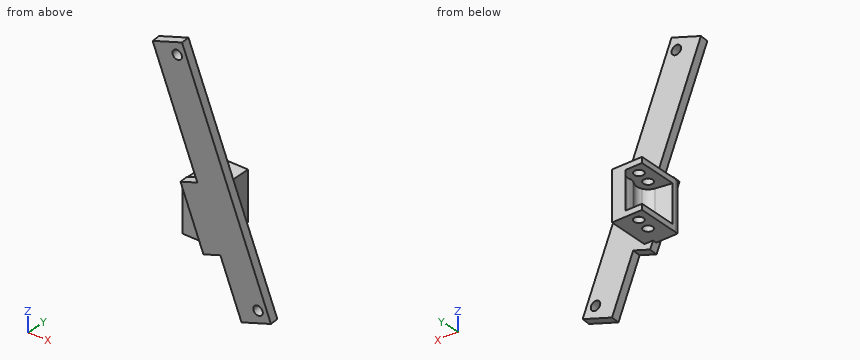
from build123d import *

# Parameters (mm, degrees)
BOSS_EXTRUDE1_DEPTH = 29.21
SKETCH2_R           = 3.175
BOSS_EXTRUDE2_DEPTH = 3.81
SKETCH3_R           = 3.175
BOSS_EXTRUDE3_DEPTH = 3.81
SKETCH4_R           = 3.175
BOSS_EXTRUDE4_DEPTH = 5.588
BOSS_EXTRUDE5_DEPTH = 33.02


with BuildPart() as part:
    # Sketch1 → Boss-Extrude1 (new body)
    with BuildSketch(Plane.XY):
        with BuildLine():
            Line((468.75530918, 278.776071532), (459.631228606, 278.776071532))
            ThreePointArc((459.631228606, 278.776071532), (460.543620658, 278.201967285), (461.366897066, 277.506071532))
            ThreePointArc((461.366897066, 277.506071532), (463.397272377, 274.114329254), (463.477224231, 270.162121354))
            ThreePointArc((463.477224231, 270.162121354), (463.399405765, 268.135304283), (464.120754615, 266.239598875))
            ThreePointArc((464.120754615, 266.239598875), (465.307742726, 262.469481888), (464.467858916, 258.607187485))
            ThreePointArc((464.467858916, 258.607187485), (462.151375158, 255.897407535), (458.862647092, 254.521445295))
            Line((458.862647092, 254.521445295), (448.43530918, 252.810420021))
            Line((448.43530918, 252.810420021), (448.43530918, 250.486101833))
            Line((448.43530918, 250.486101833), (468.75530918, 250.486101833))
            Line((468.75530918, 250.486101833), (468.75530918, 278.776071532))
        make_face()
    extrude(amount=-BOSS_EXTRUDE1_DEPTH)

    # Sketch2 → Boss-Extrude2 (add)
    with BuildSketch(Plane.XY):
        Polygon((448.43530918, 252.810420021), (448.43530918, 278.776071532), (468.75530918, 278.776071532), (468.75530918, 250.486101833), (448.43530918, 250.486101833), align=None)
        with Locations(Location((455.996603091, 271.987703521, 0), (0, 0, 180))):
            Circle(SKETCH2_R, mode=Mode.SUBTRACT)
        with Locations(Location((457.615851502, 262.119672583, 0), (0, 0, 180))):
            Circle(SKETCH2_R, mode=Mode.SUBTRACT)
    extrude(amount=BOSS_EXTRUDE2_DEPTH)

    # Sketch3 → Boss-Extrude3 (add)
    # profile 1 of 3: a face of its own
    with BuildSketch(Plane(origin=(0, 0, -25.4), x_dir=(-1, 0, 0), z_dir=(0, 0, -1))):
        with BuildLine():
            Line((-464.467858916, 258.607187485), (-448.43530918, 255.976401177))
            Line((-448.43530918, 255.976401177), (-448.43530918, 275.384123064))
            Line((-448.43530918, 275.384123064), (-461.366897066, 277.506071532))
            ThreePointArc((-461.366897066, 277.506071532), (-463.397272377, 274.114329254), (-463.477224231, 270.162121354))
            ThreePointArc((-463.477224231, 270.162121354), (-463.399405765, 268.135304283), (-464.120754615, 266.239598875))
            ThreePointArc((-464.120754615, 266.239598875), (-465.307742726, 262.469481888), (-464.467858916, 258.607187485))
        make_face()
        with Locations((-457.615851502, 262.119672583)):
            Circle(SKETCH3_R, mode=Mode.SUBTRACT)
        with Locations((-455.996603091, 271.987703521)):
            Circle(SKETCH3_R, mode=Mode.SUBTRACT)
    # profile 2 of 3: a face of its own
    with BuildSketch(Plane(origin=(0, 0, -25.4), x_dir=(-1, 0, 0), z_dir=(0, 0, -1))):
        with BuildLine():
            Line((-458.862647092, 254.521445295), (-448.43530918, 252.810420021))
            Line((-448.43530918, 252.810420021), (-448.43530918, 255.976401177))
            Line((-448.43530918, 255.976401177), (-464.467858916, 258.607187485))
            ThreePointArc((-464.467858916, 258.607187485), (-462.151375158, 255.897407535), (-458.862647092, 254.521445295))
        make_face()
    # profile 3 of 3: a face of its own
    with BuildSketch(Plane(origin=(0, 0, -25.4), x_dir=(-1, 0, 0), z_dir=(0, 0, -1))):
        with BuildLine():
            Line((-461.366897066, 277.506071532), (-448.43530918, 275.384123064))
            Line((-448.43530918, 275.384123064), (-448.43530918, 278.776071532))
            Line((-448.43530918, 278.776071532), (-459.631228606, 278.776071532))
            ThreePointArc((-459.631228606, 278.776071532), (-460.543620658, 278.201967285), (-461.366897066, 277.506071532))
        make_face()
    extrude(amount=BOSS_EXTRUDE3_DEPTH)

    # Sketch4 → Boss-Extrude4 (add)
    with BuildSketch(Plane(origin=(-3.84203447, 241.841104975, 11.406767954), x_dir=(0.9998741117550617, 0.015849347043774307, 0.0007475562269394091), z_dir=(-0.015866967007794316, 0.9987637706378837, 0.04710806533037044))):
        Polygon((459.215763784, -85.500450968), (512.667124492, 73.389830794), (492.808231658, 80.070446074), (480.07788451, 42.228033485), (468.640206694, 46.075716527), (454.8306113, 5.025115122), (466.268289117, 1.17743208), (439.35687095, -78.819835688), align=None)
        with Locations(Location((455.674707496, -76.269609027, 0), (0, 0, 270))):
            Circle(SKETCH4_R, mode=Mode.SUBTRACT)
        with Locations(Location((504.266853595, 68.176101666, 0), (0, 0, 270))):
            Circle(SKETCH4_R, mode=Mode.SUBTRACT)
    extrude(amount=-BOSS_EXTRUDE4_DEPTH)

    # Sketch5 → Boss-Extrude5 (add)
    with BuildSketch(Plane.XY.offset(3.81)):
        Polygon((468.75530918, 250.486101833), (448.560469366, 250.486101833), (448.560469366, 248.52896412), (468.75530918, 248.393245925), align=None)
    extrude(amount=-BOSS_EXTRUDE5_DEPTH)


solid = part.part
Check sheet for the modelled part. Datum: model origin and axes. Units: mm. Give positions to 0.01 mm unless a question says otherwise; leave off trailing zeros. Write each loop counter-clockwise with the first axis right and the second up, starting at its lowest first coordinate (ties: lowest second). Pieces come first, ordered by that corner, then holes. Notation, with made-up numbers: (-15.5, 73) -> (15.5, 73) arc R28 ccw to (15.5, 101) -> close; hole circle Ø2 at (88, 73.5). An arc over 180 degrees is marked (long way). Use one line per item in the form item = value. Start each with the question number.
1. Section check A-A (x = 443). Record the cut outline in (y, z), and give its area (3 significant figures).
2. Go/stop test with flat-tipped pins: P1, Ø8.5, axis at x = 456.5, y = 261, coming from the -Z side; P2, Ø8, axis at x = 454, z = 36.5, coming from the -Y side; P3, Ø12, axis at x = 465, z = 64, coming from the +Y side; P4, Ø12, axis at x = 457.5, y = 244, coming from the +Z side. Record where each tip stops, or that it passes through.
3. Section check B-B (z = 74). Record the cut outline in (x, y), and give its area (3 significant figures).
4. Thickness scan on line 1 along Z through (x, y) = (457, 267); line 2 along X through (y, z) = (252, -5); line 3 along X through (y, z) = (247, -41.5). Record the ranges inside material, lowest first. Write a range as from..to.
Conclusion:
q1.outline = (239.51, 92.71) -> (240.67, 68.08) -> (246.27, 68.08) -> (245.09, 93.01) -> close
q1.area = 139 mm²
q2.P1 = -29.21
q2.P2 = 242.14
q2.P3 = 247.11
q2.P4 = 97.16
q3.outline = (441.01, 240.36) -> (463.12, 240.71) -> (463.12, 246.31) -> (441.01, 245.96) -> close
q3.area = 124 mm²
q4.line_1 = -29.21..-25.4, 0..3.81
q4.line_2 = 448.44..468.76
q4.line_3 = 479.91..502.02
